Drawing for the job (mm, zero at the part's lowest x, y, z). Give positions to 0.01 mm unless a question says otherwise; leave off trailing zeros. Loops run counter-clockwise (first coordinate to the right, second up) from the corner with the lowest first, then second, coordinate; pieces in that order, holes last. Notation, with made-up numbers: (23.25, 67.5) -> (42.25, 67.5) arc R24 cw to (42.25, 90.5) -> close; hole circle Ø4 at (-15.75, 48.5). An arc over 180 degrees is marked (long way). Write item = value, one per line.
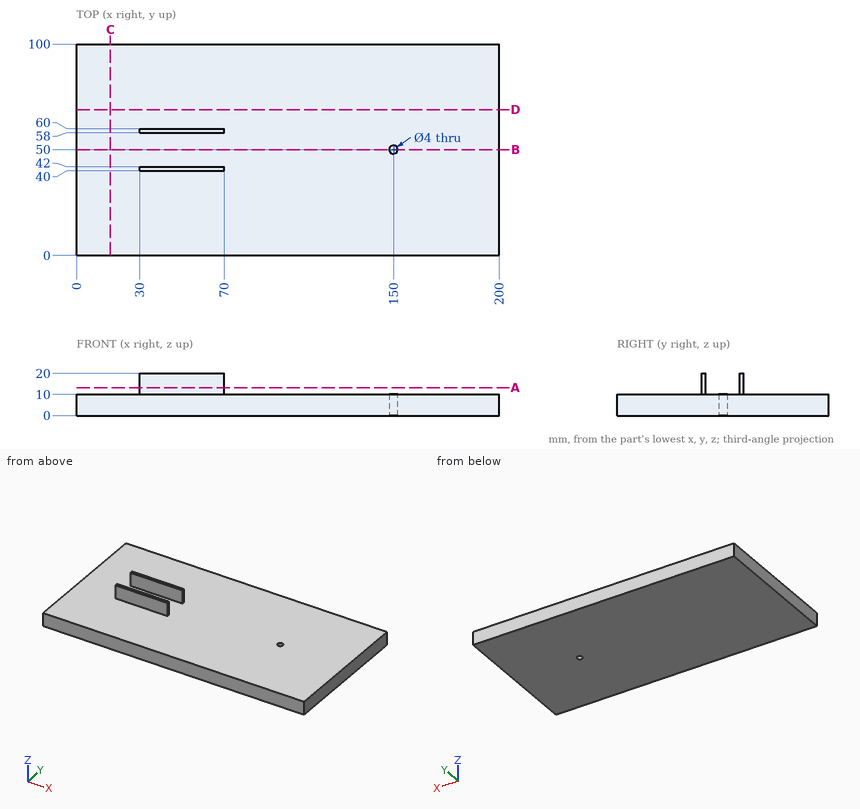
1) Slice it at D-D, the plane y = 69. List the corners of the cut face in (x, z), and give its area (3 significant figures).
Resolved:
outline = (0, 0) -> (200, 0) -> (200, 10) -> (0, 10) -> close
area = 2,000 mm²
2) Drill centre lines: line 1 along Y through (x, z) = (150, 4.5); line 2 along Y through (x, z) = (32.5, 14.75); line 3 along Z through (x, y) = (94, 22.5). Where is each one in solid material? Low to high. Write a range as [from, to].
Resolved:
line_1 = [0, 48], [52, 100]
line_2 = [40, 42], [58, 60]
line_3 = [0, 10]
3) Drop flat-ended pins along their axis: P1, Ø3, axis at y = 63.5, z = 12.5, coming from the +X side (3 decimals); P2, Ø1.6, axis at y = 58.5, z = 14, coming from the -X side; P3, Ø8, axis at x = 44, z = 15.5, coming from the -Y side; P4, Ø2, axis at x = 146, y = 31.5, coming from the +Z side. Give the stop position or say it passes through.
Resolved:
P1 = through
P2 = 30
P3 = 40
P4 = 10
4) Slice it at B-B, the plane y = 50. List the corners of the cut face in (x, z).
Resolved:
outline = (0, 0) -> (148, 0) -> (148, 10) -> (0, 10) -> close; (152, 0) -> (200, 0) -> (200, 10) -> (152, 10) -> close
5) Slice it at C-C, the plane x = 16. List the corners of the cut face in (y, z).
Resolved:
outline = (0, 0) -> (100, 0) -> (100, 10) -> (0, 10) -> close
6) Slice it at A-A, the plane z = 13.25. List the corners of the cut face in (x, y).
Resolved:
outline = (30, 40) -> (70, 40) -> (70, 42) -> (30, 42) -> close; (30, 58) -> (70, 58) -> (70, 60) -> (30, 60) -> close
